from build123d import *

# Parameters (mm, degrees)
SKETCH1_R           = 1.4224
SKETCH1_R_2         = 3.175
SKETCH1_R_3         = 3.048
BOSS_EXTRUDE2_DEPTH = 4.318


with BuildPart() as part:
    # Sketch1 → Boss-Extrude2 (new body)
    with BuildSketch(Plane(origin=(0, 0, 0), x_dir=(1, 0, 0), z_dir=(0, 1, 0))):
        Polygon((0, 20.32), (0, 100), (100, 100), (100, 20.32), (142.418, 20.32), (142.418, 0), (100, 0), (25.4, 0), (25.4, -25.4), (0, -25.4), (0, 0), (-42.418, 0), (-42.418, 20.32), align=None)
        with Locations((2.8448, 2.8448)):
            Circle(SKETCH1_R, mode=Mode.SUBTRACT)
        with Locations((97.1552, 2.8448)):
            Circle(SKETCH1_R, mode=Mode.SUBTRACT)
        with Locations((2.8448, 97.1552)):
            Circle(SKETCH1_R, mode=Mode.SUBTRACT)
        with Locations((97.1552, 97.1552)):
            Circle(SKETCH1_R, mode=Mode.SUBTRACT)
        with Locations((12.7, -23.2664)):
            Circle(SKETCH1_R, mode=Mode.SUBTRACT)
        with Locations((12.7, -2.1336)):
            Circle(SKETCH1_R, mode=Mode.SUBTRACT)
        with Locations((-6.985, 10.16)):
            Circle(SKETCH1_R_2, mode=Mode.SUBTRACT)
        with Locations((-35.433, 10.16)):
            Circle(SKETCH1_R_2, mode=Mode.SUBTRACT)
        with Locations((106.985, 10.16)):
            Circle(SKETCH1_R_3, mode=Mode.SUBTRACT)
        with Locations((135.433, 10.16)):
            Circle(SKETCH1_R_2, mode=Mode.SUBTRACT)
    extrude(amount=BOSS_EXTRUDE2_DEPTH)


solid = part.part
Could you check a few things on this model? Use its own coordinates, in mm. A direction names the side the tool comes from. Give positions to 0.01 mm unless a question says otherwise; leave off trailing zeros. Order: outer loops, then holes, each group sorted by start corner. A loop starts at its lowest first (then second) coordinate and runs counter-clockwise, first axis right, second up.
1. Suppose I cut it at C-C (x = -22). Write out the boundary of the cut face in (y, z), plus the area to 3 significant figures.
Answers below:
outline: (0, -20.32) - (4.32, -20.32) - (4.32, 0) - (0, 0) - close
area: 87.7 mm2
2. I need wall thicknesses on L1, parallel to Z at x = 12.7, y = 2.9; L2, parallel to X at y = 1.75, z = -10.16; L3, parallel to Z at x = -7, y = 1.7. Which ranges of each line are inside material? Lowest first, please.
Answers below:
L1: z = -100 to 0.71, 3.56 to 21.84, 24.69 to 25.4
L2: x = -42.42 to -38.61, -32.26 to -10.16, -3.81 to 103.94, 110.03 to 132.26, 138.61 to 142.42
L3: z = -20.32 to -13.33, -6.99 to 0
3. Suppose I cut it at D-D (z = -89). Write out the boundary of the cut face in (x, y).
Answers below:
outline: (0, 0) - (100, 0) - (100, 4.32) - (0, 4.32) - close
4. For pin 1 (1.3 mm diameter, centred on x = -15, y = 1.5, fed in from +Z); pin 2 (4.5 mm diameter, centred on x = 2.84, z = -97.16, fed in from +Y); pin 3 (2 mm diameter, centred on x = 124, y = 1.5, fed in from -Z); pin 4 (1.5 mm diameter, centred on y = 2.5, z = -48.5, fed in from -X), each with a flat end and sliding along its axis, tell me the tip position at first contact or that it passes through.
Answers below:
pin 1: stops at z = 0
pin 2: stops at y = 4.32
pin 3: stops at z = -20.32
pin 4: stops at x = 0
5. Which directions (+Z, -Z, +X, -X, +Y, -Y) give clear straight access to the entire face, cutting with the end or side of a thin tool? Please do faces 5 (the flat face through (142.418, 2, -10)), 6 (the flat face through (-22, 2, -20.32)), 7 (the flat face through (51, 4.318, -52)), 8 (the flat face through (0, 2, 13)), 9 (the flat face through (83, 2, 0)).
Answers below:
face 5: +Z, -Z, +X, +Y, -Y
face 6: -Z, -X, +Y, -Y
face 7: +Z, -Z, +X, -X, +Y
face 8: +Z, -X, +Y, -Y
face 9: +Z, +X, +Y, -Y
6. Thinking about a two-plate mould opening in X: for faces 1 (the flat face through (100, 2, -61)), 2 (the flat face through (121, 2, -20.32)), 3 (the flat face through (0, 2, -60)), 4 (the cylindrical face through (-9.325, 2.129, -12.306)), which applies, +X half, -X half, draft (parallel to the pull), parting line (faces both ways), or undercut?
Answers below:
face 1: +X half
face 2: draft
face 3: -X half
face 4: undercut
7. Suppose I cut it at B-B (y = 1.3). State how many separate pieces and enclosed holes the cut face has, plus the area to 3 significant figures.
Answers below:
separate pieces: 1
enclosed holes: 10
area: 12,200 mm2
8. Suppose I cut it at A-A (z = -10.16). Write out the boundary of the cut face in (x, y).
Answers below:
outline: (-42.42, 0) - (-38.61, 0) - (-38.61, 4.32) - (-42.42, 4.32) - close; (-32.26, 0) - (-10.16, 0) - (-10.16, 4.32) - (-32.26, 4.32) - close; (-3.81, 0) - (103.94, 0) - (103.94, 4.32) - (-3.81, 4.32) - close; (110.03, 0) - (132.26, 0) - (132.26, 4.32) - (110.03, 4.32) - close; (138.61, 0) - (142.42, 0) - (142.42, 4.32) - (138.61, 4.32) - close
